Build history of the part. All positions in model axes, mm. A direction names the side the tool comes from. Give positions to 0.01 mm unless a question says otherwise; leave off trailing zeros. Order: outer loops, then holes, each group sorted by start corner. A loop starts at its lowest first (then second) coordinate and runs counter-clockwise, first axis right, second up. Notation, with made-up numbers: M -40,-4.5 L -6,-4.5 A25 cw -6,30.5 Z; hole C -4.75,72 d6. An arc over 180 degrees is marked long. Answer as CSV lines item,"result".
from build123d import *

# Parameters (mm, degrees)
EXTRUDE_1_DEPTH = 2
SKETCH_2_R      = 2
EXTRUDE_2_DEPTH = 2
SKETCH_3_R      = 3
EXTRUDE_4_DEPTH = 15


with BuildPart() as part:
    # 草图1 → 凸台-拉伸1 (new body)
    with BuildSketch(Plane.XY):
        with BuildLine():
            Line((-25, 5), (15, 5))
            ThreePointArc((15, 5), (20, 0), (15, -5))
            Line((15, -5), (-25, -5))
            ThreePointArc((-25, -5), (-30, 0), (-25, 5))
        make_face()
    extrude(amount=EXTRUDE_1_DEPTH)

    # 草图2 → 凸台-拉伸2 (add)
    with BuildSketch(Plane(origin=(0, 0, 0), x_dir=(-1, 0, 0), z_dir=(0, 0, -1))):
        with Locations((25, 0)):
            Circle(SKETCH_2_R)
    extrude(amount=EXTRUDE_2_DEPTH)

    # 草图3 → 凸台-拉伸4 (add)
    with BuildSketch(Plane(origin=(0, 0, 0), x_dir=(-1, 0, 0), z_dir=(0, 0, -1))):
        with Locations((-15, 0)):
            Circle(SKETCH_3_R)
    extrude(amount=-EXTRUDE_4_DEPTH)


solid = part.part
Item 1: Drop flat-ended pins along their axis: pin 1 (3 mm diameter, centred on x = 11.5, y = 1, fed in from -Z); pin 2 (5 mm diameter, centred on x = 5, y = -1.5, fed in from +Z); pin 3 (3 mm diameter, centred on y = -3, z = 3, fed in from +X). Give the stop position or say it passes through.
Geometry says:
pin 1,"stops at z = 0"
pin 2,"stops at z = 2"
pin 3,"stops at x = 19.63"
Item 2: Band-saw the part on B-B (z = 0.75). Give the cut face in (x, y), and give its area (3 significant figures).
Geometry says:
outline,"M -25,-5 L 15,-5 A5 ccw 15,5 L -25,5 A5 ccw Z"
area,"479 mm2"
Item 3: Band-saw the part on C-C (y = -2.5). Give the cut face in (x, z), and give its area (3 significant figures).
Geometry says:
outline,"M -29.33,0 L 19.33,0 L 19.33,2 L 16.66,2 L 16.66,15 L 13.34,15 L 13.34,2 L -29.33,2 Z"
area,"140 mm2"
Item 4: Pull direction Z, two halves, no side cores. Call faces 3 (the flat face through (-25, 0, -2)), 4 (the cylindrical face through (-23, 0, -1)), 5 (the flat face through (15, 0, 15)): released by +Z, released by -Z, zero draft, split by the parting line, or undercut.
Geometry says:
face 3,"released by -Z"
face 4,"zero draft"
face 5,"released by +Z"
Item 5: 3-axis set-ups, long thin cutter, end or side, ignore diameter. For faces 1 (the flat face through (-5, 5, 1)), 2 (the cylindrical face through (18, 0, 8)): which of +Z, -Z, +X, -X, +Y, -Y reach the whole face in a straight line?
Geometry says:
face 1,"+Z, -Z, +X, -X, +Y"
face 2,"+Z"
Item 6: Band-saw the part on D-D (z = 12.5). Give the cut face in (x, y), and give its area (3 significant figures).
Geometry says:
outline,"C 15,0 d6"
area,"28.3 mm2"
Item 7: Band-saw the part on A-A (x = -24). Give the cut face in (y, z).
Geometry says:
outline,"M -5,0 L -1.73,0 L -1.73,-2 L 1.73,-2 L 1.73,0 L 5,0 L 5,2 L -5,2 Z"
Item 8: Probe line 1 along Z through (x, y) = (4.5, -3.5); line 2 along Z through (x, y) = (17, -2); line 3 along X through (y, z) = (-0.5, 14.25). List the from-to ranges inside material, lowest first. Write a range as from..to.
Geometry says:
line 1,"z = 0..2"
line 2,"z = 0..15"
line 3,"x = 12.04..17.96"
